For this review, take the finished solid that the model builds, in its own axes (mm). Give positions to 0.01 mm unless a question says otherwise; leave off trailing zeros. Write each loop counter-clockwise with the first axis right and the second up, starting at its lowest first coordinate (ties: lowest second). Pieces come first, ordered by that corner, then holes. Notation, with made-up numbers: (47, 10) -> (87, 10) arc R21 cw to (87, 19) -> close; hole circle Ø5 at (16, 32). An arc over 180 degrees is marked (long way). Return JSON: item names as keys, results as strings.
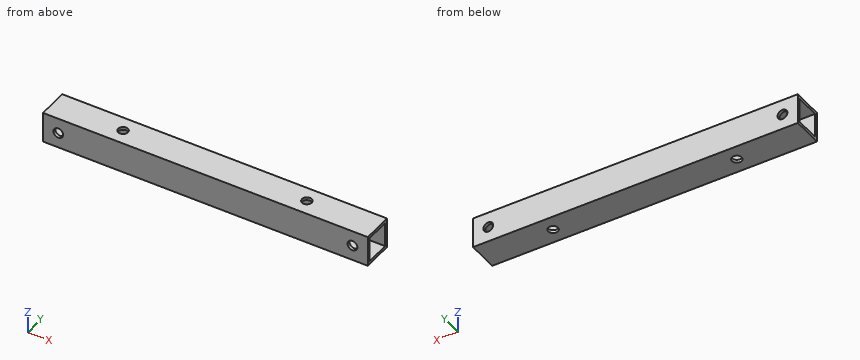
Autodesk Inventor part; units mm, degrees
ref_plane "YZ Plane" through (0, 0, 0) normal (1, 0, 0) x (0, 1, 0)
ref_plane "XZ Plane" through (0, 0, 0) normal (0, 1, 0) x (-1, 0, 0)
ref_plane "XY Plane" through (0, 0, 0) normal (0, 0, 1) x (1, 0, 0)
sketch "スケッチ1" plane through (0, 0, 0) normal (1, 0, 0) x (0, 1, 0)
  line L0 (0, 0) -> (10, 0)
  line L1 (10, 0) -> (10, -10)
  line L2 (10, -10) -> (0, -10)
  line L3 (0, -10) -> (0, 0)
  line L4 (1, -1) -> (9, -1)
  line L5 (9, -1) -> (9, -9)
  line L6 (9, -9) -> (1, -9)
  line L7 (1, -9) -> (1, -1)
  dimension "d0" = 10
  dimension "d1" = 10
  dimension "d2" = 8
  dimension "d3" = 8
  dimension "d4" = 1
  dimension "d5" = 1
extrude "押し出し1" add sketch "スケッチ1" along normal blind 106
sketch "スケッチ2" plane through (0, 10, 0) normal (0, 1, 0) x (1, 0, 0)
  line L0 (0, 9) -> (0, 1)
  line L1 (0, 5) -> (120, 5)
  line L2 (106, 10) -> (106, 0)
  point P0 (0, 0)
  point P1 (5, 5)
  point P2 (101, 5)
  dimension "d8" = 5
  dimension "d9" = 5
hole "穴1" at (5, 10, -5) at (101, 10, -5) direction (0, -1, 0) diameter 3.2 end through all
sketch "スケッチ3" plane through (0, 0, 0) normal (0, 0, 1) x (1, 0, 0)
  line L0 (0, 0) -> (0, 10)
  line L1 (0, 5) -> (106, 5)
  line L2 (106, 0) -> (106, 10)
  point P0 (23, 5)
  point P1 (83, 5)
  point P2 (53, 5)
  dimension "d17" = 30
  dimension "d18" = 30
hole "穴2" at (23, 5, 0) at (83, 5, 0) direction (0, 0, -1) diameter 3.2 end through all
properties part number "link2_pipe3" material "アルミニウム 6061"
1. Add section C-C, the plane x = 83. State the section outline as (y, z) points, plus the area to 3 significant figures.
Results found:
{"outline": "(0, -10) -> (3.4, -10) -> (3.4, -9) -> (1, -9) -> (1, -1) -> (3.4, -1) -> (3.4, 0) -> (0, 0) -> close; (6.6, -10) -> (10, -10) -> (10, 0) -> (6.6, 0) -> (6.6, -1) -> (9, -1) -> (9, -9) -> (6.6, -9) -> close", "area": "29.6 mm²"}
2. To check wall thickness, follow probe 1 along X at (y, z) = (0.35, -5); probe 2 along X at (y, z) = (5, -9.55); probe 3 along Z at (x, y) = (84, 2.75). State the ranges of each line that lie inside material, in increasing order.
Results found:
{"probe 1": "x = 0 to 3.4, 6.6 to 99.4, 102.6 to 106", "probe 2": "x = 0 to 21.4, 24.6 to 81.4, 84.6 to 106", "probe 3": "z = -10 to -9, -1 to 0"}
3. Add section D-D, the plane x = 30. State the section outline as (y, z) points.
Results found:
{"outline": "(0, -10) -> (10, -10) -> (10, 0) -> (0, 0) -> close; hole (1, -9) -> (9, -9) -> (9, -1) -> (1, -1) -> close"}
4. Add section B-B, the plane z = -5. State the section outline as (x, y) points, plus the area to 3 significant figures.
Results found:
{"outline": "(0, 0) -> (3.4, 0) -> (3.4, 1) -> (0, 1) -> close; (0, 9) -> (3.4, 9) -> (3.4, 10) -> (0, 10) -> close; (6.6, 0) -> (99.4, 0) -> (99.4, 1) -> (6.6, 1) -> close; (6.6, 9) -> (99.4, 9) -> (99.4, 10) -> (6.6, 10) -> close; (102.6, 0) -> (106, 0) -> (106, 1) -> (102.6, 1) -> close; (102.6, 9) -> (106, 9) -> (106, 10) -> (102.6, 10) -> close", "area": "199 mm²"}
5. Add section A-A, the plane y = 5. State the section outline as (x, z) points, plus the area to 3 significant figures.
Results found:
{"outline": "(0, -10) -> (21.4, -10) -> (21.4, -9) -> (0, -9) -> close; (0, -1) -> (21.4, -1) -> (21.4, 0) -> (0, 0) -> close; (24.6, -10) -> (81.4, -10) -> (81.4, -9) -> (24.6, -9) -> close; (24.6, -1) -> (81.4, -1) -> (81.4, 0) -> (24.6, 0) -> close; (84.6, -10) -> (106, -10) -> (106, -9) -> (84.6, -9) -> close; (84.6, -1) -> (106, -1) -> (106, 0) -> (84.6, 0) -> close", "area": "199 mm²"}
